Input: part model. Units: mm. Frame: model coordinates. Face numbers are marked on the shaded views. A direction names the side the tool comes from. Round coordinates to 2 decimals unless told otherwise and drop trailing zeros. Order: outer loops, then holes, each group sorted by start corner. A loop starts at its lowest first (then second) coordinate and runs counter-clockwise, first axis right, second up. Notation, with made-up numbers: (21, 4.25) -> (26, 4.25) arc R31 cw to (26, 35.25) -> close; hole circle Ø6 at (-17, 83). An arc over 180 degrees is marked (long way). Use a Markdown table: item, result.
Autodesk Fusion 360 part; units mm, degrees
sketch "Sketch1" plane through (0, 0, 0) normal (0, 0, 1) x (1, 0, 0)
  line L0 (-16.0699, 13.472) -> (-6.0699, 13.472)
  line L1 (-6.0699, 13.472) -> (-6.0699, 9.472)
  line L2 (-6.0699, 9.472) -> (-16.0699, 9.472)
  line L3 (-16.0699, 9.472) -> (-16.0699, 13.472)
  dimension "d1" = 10
  dimension "d2" = 4
extrude "Extrude1" add sketch "Sketch1" along normal blind 1
sketch "Sketch2" plane through (0, 0, 1) normal (0, 0, 1) x (1, 0, 0)
  line L0 (-16.0699, 9.472) -> (-6.0699, 9.472)
  line L1 (-6.0699, 9.472) -> (-6.0699, 13.472)
  line L2 (-6.0699, 13.472) -> (-16.0699, 13.472)
  line L3 (-16.0699, 13.472) -> (-16.0699, 9.472)
  line L4 (-16.0699, 13.472) -> (-6.0699, 13.472)
  line L5 (-6.0699, 13.472) -> (-6.0699, 12.472)
  line L6 (-6.0699, 12.472) -> (-16.0699, 12.472)
  line L7 (-16.0699, 12.472) -> (-16.0699, 13.472)
  dimension "d5" = 1
  dimension "d6" = 10
extrude "Extrude2" add sketch "Sketch2" along normal blind 3 contours L1 L2 L3 L4 L5 L6 L7
fillet "Fillet1" radius 1 1 edges at (-6.0699, 9.472, 0.5)
fillet "Fillet2" radius 1 1 edges at (-16.0699, 9.472, 0.5)
fillet "Fillet3" radius 1 1 edges at (-16.0699, 12.972, 4)
fillet "Fillet4" radius 1 1 edges at (-6.0699, 12.972, 4)
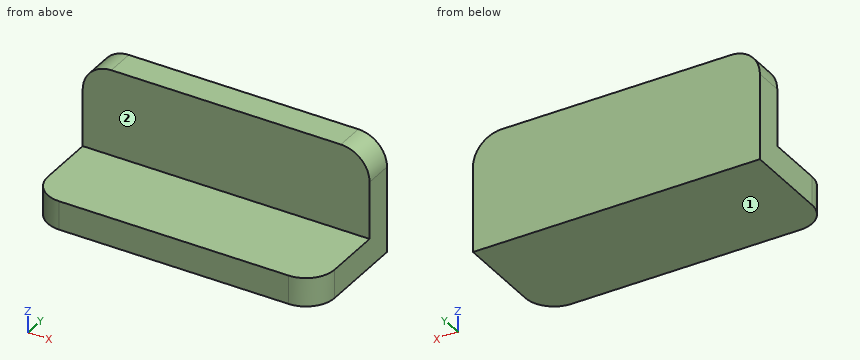
1) Cut plane B-B on y = 11.1. Return loops of the section in (x, z), and give its area (3 significant figures).
Answer key:
| item | result |
|---|---|
| outline | (-16.07, 0) -> (-6.07, 0) -> (-6.07, 1) -> (-16.07, 1) -> close |
| area | 10.0 mm^2 |
2) Set-up query: the marked faces 1 and 2. Return all of +Z, -Z, +X, -X, +Y, -Y with unobstructed straight access to the full face (end or side cutting, diameter ignored); none if empty.
Answer key:
| item | result |
|---|---|
| face 1 | -Z, +X, -X, +Y, -Y |
| face 2 | +Z, +X, -X, -Y |
3) Contact query for flat-ended pins moving along their axis: P1, Ø1.5, axis at x = -12.5, z = 3, coming from the -Y side; P2, Ø2, axis at x = -12, y = 12, coming from the -Z side. Output: stop coordinate, or through.
Answer key:
| item | result |
|---|---|
| P1 | stops at y = 12.47 |
| P2 | stops at z = 0 |
4) Cut plane A-A on x = -10.75. Return loops of the section in (y, z).
Answer key:
| item | result |
|---|---|
| outline | (9.47, 0) -> (13.47, 0) -> (13.47, 4) -> (12.47, 4) -> (12.47, 1) -> (9.47, 1) -> close |
5) Cut plane C-C on z = 2.35. Return loops of the section in (x, y).
Answer key:
| item | result |
|---|---|
| outline | (-16.07, 12.47) -> (-6.07, 12.47) -> (-6.07, 13.47) -> (-16.07, 13.47) -> close |
6) Ray query, probe 1 along Y at (x, z) = (-9.75, 2.3); probe 2 along Z at (x, y) = (-14.5, 9.7); probe 3 along Z at (x, y) = (-15.5, 12.65). Return the intervals inside material, ascending.
Answer key:
| item | result |
|---|---|
| probe 1 | y = 12.47 to 13.47 |
| probe 2 | z = 0 to 1 |
| probe 3 | z = 0 to 3.9 |
